Study the drawing (mm; zero at the part's minimum x, y, z) and answer. A direction names the side the tool comes from. Round coordinates to 2 decimals unless told otherwise and drop trailing zeros. Loops run counter-clockwise (first coordinate to the right, second up) from the corner with the lowest first, then second, coordinate; pieces in that order, holes last. Notation, with made-up numbers: (66.5, -3) -> (80.5, -3) arc R30 ccw to (80.5, 24) -> close; hole circle Ø9 at (15, 65). An arc over 180 degrees is marked (long way). Use one line per item in the form item = value.
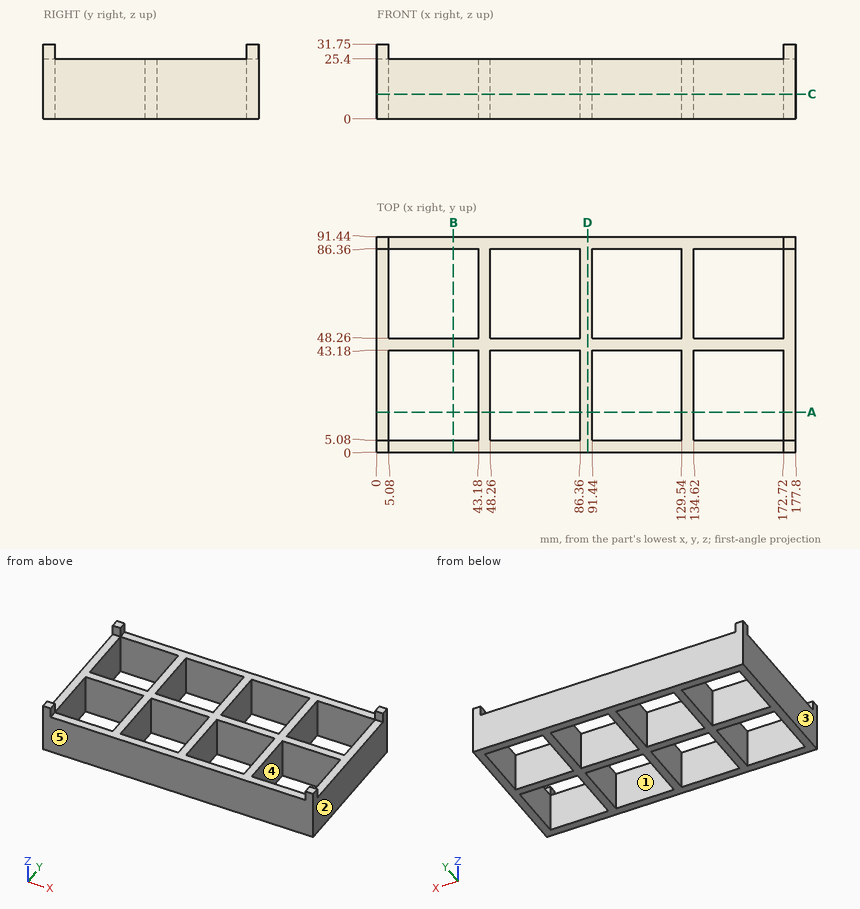
(1) Find section C-C, the plane z = 10.5. State how many separate pieces and enclosed holes the cut face has, then the cut area to 3 significant figures.
Completed:
separate_pieces = 1
enclosed_holes = 8
area = 4,650 mm2
(2) For a pull along Y with two mould halves and no side action, classify the marked faces 3, 4 and 5 as +Y half, -Y half, draft (parallel to the pull), parting line (faces both ways), or undercut.
Completed:
face_3 = draft
face_4 = undercut
face_5 = -Y half
(3) Consider L1, parallel to X at y = 17, z = 2; L2, parallel to Y at x = 135.5, z = 17; L3, parallel to Z at x = 122, y = 46. Determine where each line is inside the solid, lowest interval first.
Completed:
L1 = 0 to 5.08, 43.18 to 48.26, 86.36 to 91.44, 129.54 to 134.62, 172.72 to 177.8
L2 = 0 to 5.08, 43.18 to 48.26, 86.36 to 91.44
L3 = 0 to 25.4
(4) Find section B-B, the plane x = 32.5. Write down the section's boundary in (y, z), then the cut area to 3 significant figures.
Completed:
outline = (0, 0) -> (5.08, 0) -> (5.08, 25.4) -> (0, 25.4) -> close; (43.18, 0) -> (48.26, 0) -> (48.26, 25.4) -> (43.18, 25.4) -> close; (86.36, 0) -> (91.44, 0) -> (91.44, 25.4) -> (86.36, 25.4) -> close
area = 387 mm2
(5) For the marked faces 1 and 2, determine the directions among +Z, -Z, +X, -X, +Y, -Y from which every point of the face is accessible in a straight line to the end or side of a thin tool.
Completed:
face_1 = +Z, -Z
face_2 = +Z, -Z, +X, +Y, -Y
(6) Given P1, Ø10, axis at x = 88, y = 29.5, coming from the +Z side, flat-ended and moving along its own axis, determine where the tip first touches the part or whether it passes through.
Completed:
P1 = 25.4
(7) Find section D-D, the plane x = 89.5. Write down the section's boundary in (y, z), then the cut area to 3 significant figures.
Completed:
outline = (0, 0) -> (91.44, 0) -> (91.44, 25.4) -> (0, 25.4) -> close
area = 2,320 mm2
(8) Find section A-A, the plane y = 17. Write down the section's boundary in (x, z).
Completed:
outline = (0, 0) -> (5.08, 0) -> (5.08, 25.4) -> (0, 25.4) -> close; (43.18, 0) -> (48.26, 0) -> (48.26, 25.4) -> (43.18, 25.4) -> close; (86.36, 0) -> (91.44, 0) -> (91.44, 25.4) -> (86.36, 25.4) -> close; (129.54, 0) -> (134.62, 0) -> (134.62, 25.4) -> (129.54, 25.4) -> close; (172.72, 0) -> (177.8, 0) -> (177.8, 25.4) -> (172.72, 25.4) -> close
